The listing builds one solid part. Answer for the finished solid, in the listing's coordinates (mm). Give positions to 0.01 mm unless a question says otherwise; leave off trailing zeros. Write each loop counter-clockwise with the first axis right and the second up, starting at its lowest first coordinate (ties: lowest second). Pieces come first, ordered by that corner, then holes. Notation, with made-up numbers: (4.25, -10) -> (34.25, -10) arc R20 ccw to (34.25, 10) -> close; hole circle Ø4 at (33.5, 24). An arc over 180 degrees is marked (long way). One line per question, with ' | ' between items.
from build123d import *

# Parameters (mm, degrees)
SKETCH1_W           = 458
SKETCH1_H           = 245
BOSS_EXTRUDE1_DEPTH = 3
CUT_EXTRUDE1_DEPTH  = 260.723410574
SKETCH3_R           = 2.5
CUT_EXTRUDE2_DEPTH  = 260.723410574
SKETCH4_R           = 11.5
CUT_EXTRUDE3_DEPTH  = 260.723410574
SKETCH5_W           = 428
SKETCH5_H           = 29
CUT_EXTRUDE4_DEPTH  = 260.723410574
SKETCH8_R           = 1.5
SKETCH8_W           = 69.9
SKETCH8_H           = 41.2
CUT_EXTRUDE5_DEPTH  = 260.723410574


with BuildPart() as part:
    # Sketch1 → Boss-Extrude1 (new body)
    with BuildSketch(Plane.XY):
        Rectangle(SKETCH1_W, SKETCH1_H)
    extrude(amount=BOSS_EXTRUDE1_DEPTH)

    # Sketch2 → Cut-Extrude1 (cut, through all)
    with BuildSketch(Plane.XY.offset(3)):
        with BuildLine():
            Line((-148, -107.5), (-148, -122.5))
            ThreePointArc((-148, -122.5), (-155, -129.5), (-162, -122.5))
            Line((-162, -122.5), (-162, -107.5))
            ThreePointArc((-162, -107.5), (-155, -100.5), (-148, -107.5))
        make_face()
        with BuildLine():
            Line((162, -107.5), (162, -122.5))
            ThreePointArc((162, -122.5), (155, -129.5), (148, -122.5))
            Line((148, -122.5), (148, -107.5))
            ThreePointArc((148, -107.5), (155, -100.5), (162, -107.5))
        make_face()
    extrude(amount=-CUT_EXTRUDE1_DEPTH, mode=Mode.SUBTRACT)

    # Sketch3 → Cut-Extrude2 (cut, through all)
    with BuildSketch(Plane.XY.offset(3)):
        with Locations((-194, 112.5)):
            Circle(SKETCH3_R)
        with Locations((-194, -107.5)):
            Circle(SKETCH3_R)
        with Locations((194, -107.5)):
            Circle(SKETCH3_R)
        with Locations((194, 112.5)):
            Circle(SKETCH3_R)
        with Locations((-215, 0)):
            Circle(SKETCH3_R)
        with Locations((-215, -90)):
            Circle(SKETCH3_R)
        with Locations((-215, 90)):
            Circle(SKETCH3_R)
        with Locations((215, 0)):
            Circle(SKETCH3_R)
        with Locations((215, -90)):
            Circle(SKETCH3_R)
        with Locations((215, 90)):
            Circle(SKETCH3_R)
        with Locations((0, 112.5)):
            Circle(SKETCH3_R)
        with Locations((0, -107.5)):
            Circle(SKETCH3_R)
    extrude(amount=-CUT_EXTRUDE2_DEPTH, mode=Mode.SUBTRACT)

    # Sketch4 → Cut-Extrude3 (cut, through all)
    with BuildSketch(Plane.XY.offset(3)):
        with Locations((-39, 91)):
            Circle(SKETCH4_R)
        with Locations((39, 91)):
            Circle(SKETCH4_R)
    extrude(amount=-CUT_EXTRUDE3_DEPTH, mode=Mode.SUBTRACT)

    # Sketch5 → Cut-Extrude4 (cut, through all)
    with BuildSketch(Plane.XY.offset(3)):
        with Locations((0, 53)):
            Rectangle(SKETCH5_W, SKETCH5_H)
    extrude(amount=-CUT_EXTRUDE4_DEPTH, mode=Mode.SUBTRACT)

    # Sketch8 → Cut-Extrude5 (cut, through all)
    with BuildSketch(Plane.XY.offset(3)):
        with Locations((5.296172264, 15.703565509)):
            Circle(SKETCH8_R)
        with Locations((5.679687501, -26.054673392)):
            Circle(SKETCH8_R)
        with Locations((-83.3, 14.88)):
            Circle(SKETCH8_R)
        with Locations((-83.367997673, -26.737946691)):
            Circle(SKETCH8_R)
        with Locations((-39, -5.5)):
            Rectangle(SKETCH8_W, SKETCH8_H)
    extrude(amount=-CUT_EXTRUDE5_DEPTH, mode=Mode.SUBTRACT)


solid = part.part
Item 1: Find section C-C (x = 101). Write down the section's boundary in (y, z).
Answers below:
outline: (-122.5, 0) -> (38.5, 0) -> (38.5, 3) -> (-122.5, 3) -> close; (67.5, 0) -> (122.5, 0) -> (122.5, 3) -> (67.5, 3) -> close
Item 2: Find section A-A (x = 155). Write down the section's boundary in (y, z).
Answers below:
outline: (-100.5, 0) -> (38.5, 0) -> (38.5, 3) -> (-100.5, 3) -> close; (67.5, 0) -> (122.5, 0) -> (122.5, 3) -> (67.5, 3) -> close
Item 3: Find section B-B (x = 40.5). Write down the section's boundary in (y, z), then the cut area to 3 significant figures.
Answers below:
outline: (-122.5, 0) -> (38.5, 0) -> (38.5, 3) -> (-122.5, 3) -> close; (67.5, 0) -> (79.6, 0) -> (79.6, 3) -> (67.5, 3) -> close; (102.4, 0) -> (122.5, 0) -> (122.5, 3) -> (102.4, 3) -> close | area: 580 mm²
Item 4: Find section D-D (z = 1.3). Count the separate pieces of the cut face and the enclosed holes in it, then the cut area to 3 significant figures.
Answers below:
separate pieces: 1 | enclosed holes: 20 | area: 95,200 mm²
Item 5: Consider line 1 (Y direction, x = -194, z = 2.25); line 2 (Y direction, x = 215, z = 2.15); line 3 (Y direction, x = -11, z = 0.3). Determine where each line is inside the solid, lowest interval first. Write a range as [from, to].
Answers below:
line 1: [-122.5, -110], [-105, 38.5], [67.5, 110], [115, 122.5] | line 2: [-122.5, -92.5], [-87.5, -2.5], [2.5, 87.5], [92.5, 122.5] | line 3: [-122.5, -26.1], [15.1, 38.5], [67.5, 122.5]
Item 6: A flat-ended cylindrical pin translates along its axis: pin 1 (3 mm diameter, centred on x = 215, y = 0, fed in from +Z). Find the tip coordinate at first contact, or state that the pin passes through.
Answers below:
pin 1: through
Item 7: Determine the mould class of faces 1 (the face through (-3, 2, 3)), 2 (the face through (-41.493, 79.773, 1.521)) for opening direction Y: pulls with the +Y half, pulls with the -Y half, needs draft (parallel to the pull), parting line crosses it, or undercut.
Answers below:
face 1: needs draft | face 2: undercut
